The drawing under review shows one solid part. Ordinate dimensions are in mm from its lowest x, y, z. A direction names the side the tool comes from. Coordinates: 2 decimals unless noted, no trailing zeros. Write each loop counter-clockwise with the first axis right and the second up, starting at its lowest first coordinate (ties: lowest second). Pieces come first, ordered by that corner, then holes. Notation, with made-up numbers: (46, 15) - (97, 15) arc R33 ccw to (97, 54) - close; hole circle Ø3 at (84, 41). An arc over 180 degrees is marked (long way). Use a Markdown table: item, result.
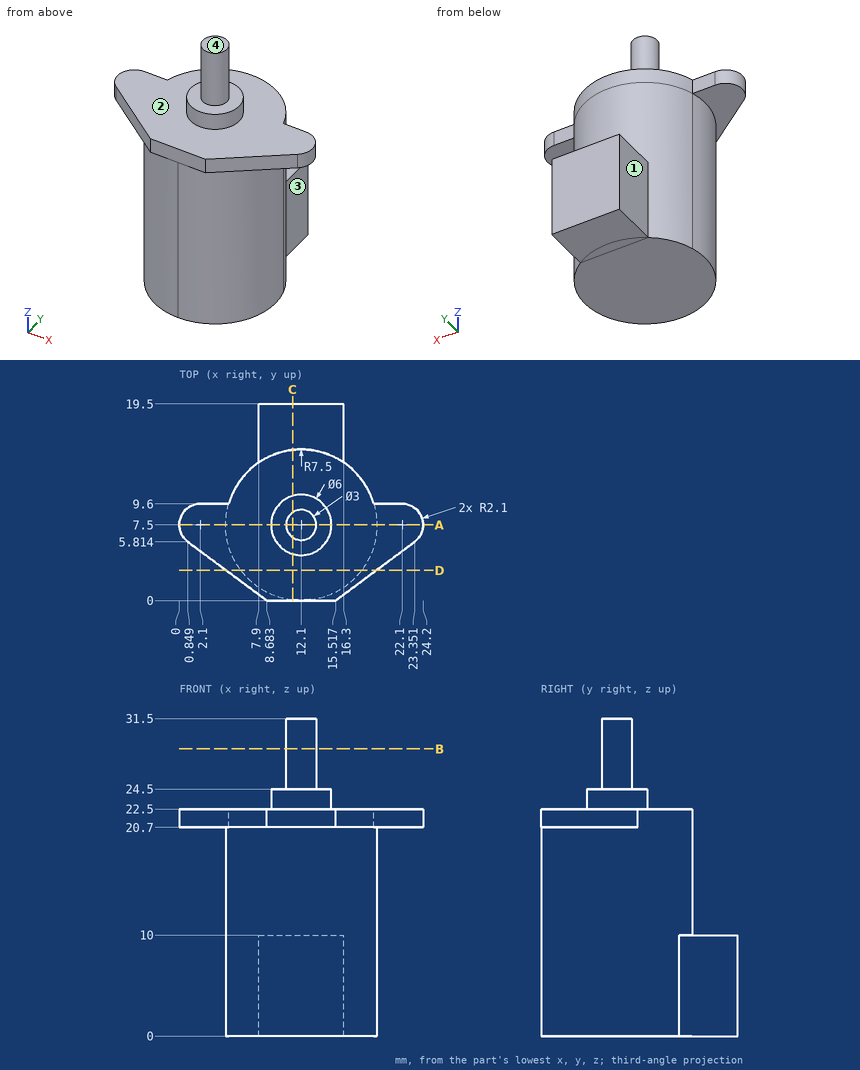
(1) Take a section at B-B on z = 28.5. Write out the cut boundary in (x, y).
Determined:
| item | result |
|---|---|
| outline | circle Ø3 at (12.1, 7.5) |
(2) Take a section at C-C on x = 11.25. Write out the cut boundary in (y, z).
Determined:
| item | result |
|---|---|
| outline | (0, 20.7) - (0.05, 20.7) - (0.05, 0) - (19.5, 0) - (19.5, 10) - (14.95, 10) - (14.95, 22.5) - (10.38, 22.5) - (10.38, 24.5) - (8.74, 24.5) - (8.74, 31.5) - (6.26, 31.5) - (6.26, 24.5) - (4.62, 24.5) - (4.62, 22.5) - (0, 22.5) - close |
(3) Take a section at D-D on y = 3. Write out the cut boundary in (x, z), and give its area (3 significant figures).
Determined:
| item | result |
|---|---|
| outline | (4.64, 20.7) - (6.1, 20.7) - (6.1, 0) - (18.1, 0) - (18.1, 20.7) - (19.56, 20.7) - (19.56, 22.5) - (4.64, 22.5) - close |
| area | 275 mm2 |
(4) Machinability: for the marked faces 1, 2, 3 and 4, which of the approach directions +Z, -Z, +X, -X, +Y, -Y give a long, thin tool a straight path to every point of the face, cutting with its end or side? Answer none if there is none.
Determined:
| item | result |
|---|---|
| face 1 | +Z, -Z, -X, +Y |
| face 2 | +Z |
| face 3 | +Z, -Z, +X, +Y |
| face 4 | +Z, +X, -X, +Y, -Y |
(5) For pin 1 (1 mm diameter, centred on y = 13, z = 15.5, fed in from +X); pin 2 (4.5 mm diameter, centred on y = 15, z = 3.5, fed in from -X) (1 decimal); pin 3 (4 mm diameter, centred on y = 13.5, z = 16, fed in from +X) (1 decimal), all flat-tipped, find the tip position at first contact; note any pin that passes through.
Determined:
| item | result |
|---|---|
| pin 1 | x = 17.69 |
| pin 2 | x = 6.7 |
| pin 3 | x = 18.4 |
(6) Take a section at A-A on y = 7.5. Write out the cut boundary in (x, z).
Determined:
| item | result |
|---|---|
| outline | (0, 20.7) - (4.6, 20.7) - (4.6, 0) - (19.6, 0) - (19.6, 20.7) - (24.2, 20.7) - (24.2, 22.5) - (15.1, 22.5) - (15.1, 24.5) - (13.6, 24.5) - (13.6, 31.5) - (10.6, 31.5) - (10.6, 24.5) - (9.1, 24.5) - (9.1, 22.5) - (0, 22.5) - close |
(7) For L1, parallel to Z at x = 5.5, y = 9.25; L2, parallel to Z at x = 21.25, y = 9; L3, parallel to X at y = 16.75, z = 3.5, list the stretches that pass through material, from the lowest coordinate up. Write a range as from..to.
Determined:
| item | result |
|---|---|
| L1 | 0..22.5 |
| L2 | 20.7..22.5 |
| L3 | 7.9..16.3 |
